```python
from build123d import *

# Parameters (mm, degrees)
SKETCH1_W           = 42.3
SKETCH1_H           = 42.3
BOSS_EXTRUDE1_DEPTH = 23.5
SKETCH2_R           = 2.05
CUT_EXTRUDE1_DEPTH  = 4.5
SKETCH3_R           = 11.4
BOSS_EXTRUDE2_DEPTH = 2
SKETCH3_3_R         = 2.5
BOSS_EXTRUDE3_DEPTH = 22
SKETCH4_W           = 16.2
SKETCH4_H           = 9.2
BOSS_EXTRUDE4_DEPTH = 5.5


with BuildPart() as part:
    # Sketch1 → Boss-Extrude1 (new body)
    with BuildSketch(Plane(origin=(0, 0, 0), x_dir=(1, 0, 0), z_dir=(0, 1, 0))):
        Rectangle(SKETCH1_W, SKETCH1_H)
    extrude(amount=-BOSS_EXTRUDE1_DEPTH)

    # Sketch2 → Cut-Extrude1 (cut)
    with BuildSketch(Plane(origin=(0, 0, 0), x_dir=(1, 0, 0), z_dir=(0, 1, 0))):
        with BuildLine():
            ThreePointArc((13.45, 15.5), (14.050431099, 14.050431099), (15.5, 13.45))
            Line((15.5, 13.45), (15.5, 15.5))
            Line((15.5, 15.5), (13.45, 15.5))
        make_face()
        with BuildLine():
            Line((15.5, 15.5), (15.5, 13.45))
            ThreePointArc((15.5, 13.45), (16.949568901, 14.050431099), (17.55, 15.5))
            ThreePointArc((17.55, 15.5), (15.5, 17.55), (13.45, 15.5))
            Line((13.45, 15.5), (15.5, 15.5))
        make_face()
        with Locations(Location((-15.5, -15.5, 0), (0, 0, 90))):
            Circle(SKETCH2_R)
        with Locations(Location((-15.5, 15.5, 0), (0, 0, 270))):
            Circle(SKETCH2_R)
        with Locations(Location((15.5, -15.5, 0), (0, 0, 270))):
            Circle(SKETCH2_R)
    extrude(amount=-CUT_EXTRUDE1_DEPTH, mode=Mode.SUBTRACT)

    # Sketch3 → Boss-Extrude2 (add)
    with BuildSketch(Plane(origin=(0, 0, 0), x_dir=(1, 0, 0), z_dir=(0, 1, 0))):
        with Locations(Location((0, 0, 0), (0, 0, 90))):
            Circle(SKETCH3_R)
    extrude(amount=BOSS_EXTRUDE2_DEPTH)

    # Sketch3_3 → Boss-Extrude3 (add)
    with BuildSketch(Plane(origin=(0, 0, 0), x_dir=(1, 0, 0), z_dir=(0, 1, 0))):
        with Locations(Location((0, 0, 0), (0, 0, 270))):
            Circle(SKETCH3_3_R)
    extrude(amount=BOSS_EXTRUDE3_DEPTH)

    # Sketch4 → Boss-Extrude4 (add)
    with BuildSketch(Plane.XY.offset(21.15)):
        with Locations((0, -18.9)):
            Rectangle(SKETCH4_W, SKETCH4_H)
    extrude(amount=BOSS_EXTRUDE4_DEPTH)


solid = part.part
```
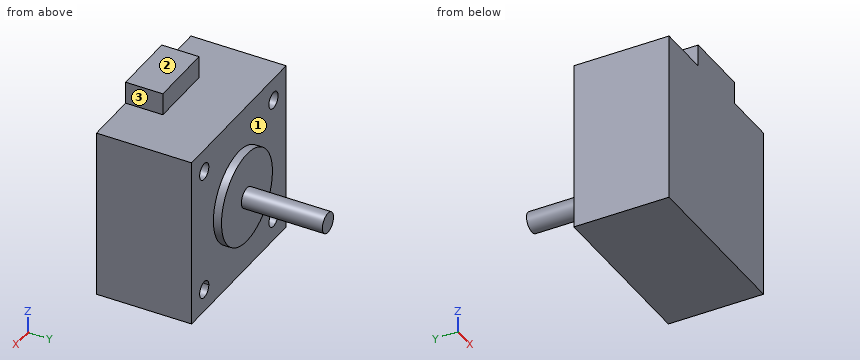
The listing builds one solid part. Answer for the finished solid, in the listing's coordinates (mm). Face numbers are marked on the shaded views. A direction names the side the tool comes from. Give positions to 0.01 mm unless a question says otherwise; leave off trailing zeros. Loops run counter-clockwise (first coordinate to the right, second up) from the corner with the lowest first, then second, coordinate; pieces in that order, holes last. Notation, with made-up numbers: (80.25, 89.5) - (127.25, 89.5) arc R19 cw to (127.25, 109.5) - close; hole circle Ø5 at (-13, 89). An arc over 180 degrees is marked (long way). Answer as CSV lines item,"result". Start each with the question number.
Item 1: For the marked faces 1, 2 and 3, determine the directions among +Z, -Z, +X, -X, +Y, -Y from which every point of the face is accessible in a straight line to the end or side of a thin tool.
Item 2: Find the intervals of material crossed by line 1 (X direction, y = -3.5, z = 15.5); line 2 (Y direction, x = -10, z = 2.5); line 3 (Y direction, x = 7, z = -17), in increasing order. Write a range as from..to.
Item 3: A cutting plane is placed at B-B on x = -15.5. Determine the outline of the cut face in (y, z), then the cut area to 3 significant figures.
Item 4: A cutting plane is placed at D-D on x = 0. Determine the outline of the cut face in (y, z).
Item 5: A cutting plane is placed at C-C on y = 15. Determine the outline of the cut face in (x, z), then the cut area to 3 significant figures.
Item 6: A cutting plane is placed at A-A on z = 15.5. Determine the outline of the cut face in (x, y), then the cut area to 3 significant figures.
Item 7: Each of these flat-tipped pins is pushed along its axis until it touches: pin 1 (3.5 mm diameter, centred on x = -15.5, z = 16, fed in from +Y); pin 2 (2 mm diameter, centred on x = -6.5, z = 1.5, fed in from +Y); pin 3 (3 mm diameter, centred on y = -17.5, z = 23.5, fed in from +X). Where does it stop, or does it pass through?
Found:
1,face 1,"+Y"
1,face 2,"+Z, +X, -X, +Y, -Y"
1,face 3,"+Z, +X, +Y, -Y"
2,line 1,"x = -21.15..-17.55, -13.45..13.45, 17.55..21.15"
2,line 2,"y = -23.5..2"
2,line 3,"y = -23.5..0"
3,outline,"(-23.5, -21.15) - (0, -21.15) - (0, -17.55) - (-4.5, -17.55) - (-4.5, -13.45) - (0, -13.45) - (0, 13.45) - (-4.5, 13.45) - (-4.5, 17.55) - (0, 17.55) - (0, 21.15) - (-23.5, 21.15) - close"
3,area,"957 mm^2"
4,outline,"(-23.5, -21.15) - (0, -21.15) - (0, -11.4) - (2, -11.4) - (2, -2.5) - (22, -2.5) - (22, 2.5) - (2, 2.5) - (2, 11.4) - (0, 11.4) - (0, 21.15) - (-14.3, 21.15) - (-14.3, 26.65) - (-23.5, 26.65) - close"
5,outline,"circle Ø5 at (0, 0)"
5,area,"19.6 mm^2"
6,outline,"(-21.15, -23.5) - (21.15, -23.5) - (21.15, 0) - (17.55, 0) - (17.55, -4.5) - (13.45, -4.5) - (13.45, 0) - (-13.45, 0) - (-13.45, -4.5) - (-17.55, -4.5) - (-17.55, 0) - (-21.15, 0) - close"
6,area,"957 mm^2"
7,pin 1,"stops at y = 0"
7,pin 2,"stops at y = 2"
7,pin 3,"stops at x = 8.1"
